The model under review builds one solid part; all positions refer to its coordinate system, in mm. A direction names the side the tool comes from. Coordinates: 2 decimals unless noted, no trailing zeros. Order: outer loops, then holes, each group sorted by start corner. A loop starts at its lowest first (then second) coordinate and runs counter-clockwise, first axis right, second up.
```python
from build123d import *

# Parameters (mm, degrees)
F1_DEPTH = 127
F2_W     = 25.4
F2_H     = 25.4
F3_DEPTH = 6.35
F4_R     = 1.397
F5_DEPTH = 25.401


with BuildPart() as f1:
    # F0 (on Front) → F1 (new body)
    with BuildSketch(Plane.XZ):
        Polygon((12.7, 12.7), (3.386421, 12.7), (3.386421, 6.477), (6.477, 6.477), (6.477, -6.477), (-6.477, -6.477), (-6.477, -4.043587), (-12.7, -4.043587), (-12.7, -12.7), (12.7, -12.7), align=None)
    extrude(amount=F1_DEPTH)

    # F2 (on face) → F3 (join)
    with BuildSketch(Plane.XZ.offset(127)):
        Rectangle(F2_W, F2_H)
    extrude(amount=F3_DEPTH)

    # F4 (on face) → F5 (cut, through all)
    with BuildSketch(Plane(origin=(-12.7, 0, 0), x_dir=(0, -1, 0), z_dir=(-1, 0, 0))):
        with Locations((130.214259, 9.271351)):
            Circle(F4_R)
    extrude(amount=-F5_DEPTH, mode=Mode.SUBTRACT)


solid = f1.part
```
(1) Wall thickness on probe 1 along X at (y, z) = (-105, -5.5); probe 2 along Z at (x, y) = (-0.5, -14.5): over which ranges is each line inside the solid? List them lowest first.
A:
probe 1: x = -12.7 to -6.48, 6.48 to 12.7
probe 2: z = -12.7 to -6.48
(2) We need section A-A, the plane y = -67. Write out the cut boundary in (x, z).
A:
outline: (-12.7, -12.7) - (12.7, -12.7) - (12.7, 12.7) - (3.39, 12.7) - (3.39, 6.48) - (6.48, 6.48) - (6.48, -6.48) - (-6.48, -6.48) - (-6.48, -4.04) - (-12.7, -4.04) - close
(3) For pin 1 Ø4 at (x, y) = (-3.5, -18) entering from +Z; pin 2 Ø1.9 at (y, z) = (-54, 9) entering from -X; pin 3 Ø5 at (x, y) = (-10.5, -58.5) entering from +Z, all flat-tipped, find the tip position at first contact; note any pin that passes through.
A:
pin 1: stops at z = -6.48
pin 2: stops at x = 3.39
pin 3: stops at z = -4.04
(4) Draft analysis for pull direction Z (two halves, no side actions). For faces 6 (the face through (-10, -63, -4.044)), 7 (the face through (0, -63, -6.477)), 8 (the face through (-12.7, -71, -8)), state which applies: released by +Z, released by -Z, zero draft, split by the parting line, or undercut.
A:
face 6: released by +Z
face 7: undercut
face 8: zero draft
(5) We need section C-C, the plane z = -2. Write out the cut boundary in (x, y).
A:
outline: (-12.7, -133.35) - (12.7, -133.35) - (12.7, 0) - (6.48, 0) - (6.48, -127) - (-12.7, -127) - close
(6) We need section B-B, the plane x = -0.25. Write out the cut boundary in (y, z).
A:
outline: (-133.35, -12.7) - (0, -12.7) - (0, -6.48) - (-127, -6.48) - (-127, 12.7) - (-133.35, 12.7) - close; hole circle Ø2.79 at (-130.21, 9.27)
(7) We need section D-D, the plane x = -8.75. Write out the cut boundary in (y, z).
A:
outline: (-133.35, -12.7) - (0, -12.7) - (0, -4.04) - (-127, -4.04) - (-127, 12.7) - (-133.35, 12.7) - close; hole circle Ø2.79 at (-130.21, 9.27)
(8) Machinability: for faces 1 (the face through (5, -63, 6.477)), 2 (the face through (6.477, -63, 0)), 3 (the face through (-6.477, -63, -5)), 4 (the face through (0, -133.35, 0)), 5 (the face through (3.386, -63, 10)), which of the approach directions +Z, -Z, +X, -X, +Y, -Y give a long, thin tool a straight path to every point of the face, cutting with its end or side? Answer none if there is none.
A:
face 1: -X, +Y
face 2: +Y
face 3: +Z, +Y
face 4: +Z, -Z, +X, -X, -Y
face 5: +Z, -X, +Y
